Read the model definition and answer for the solid it produces. Units are mm, in the model's axes. Give positions to 0.01 mm unless a question says otherwise; leave off trailing zeros. Loops run counter-clockwise (first coordinate to the right, second up) from the corner with the lowest first, then second, coordinate; pieces in that order, holes last. Notation, with made-up numbers: (18.5, 64.5) -> (22.5, 64.5) arc R18 cw to (22.5, 79.5) -> close; hole circle Ø7 at (-6.5, 56.5). An arc over 180 degrees is marked (long way). One line per item, written item: value. Start each with the question number.
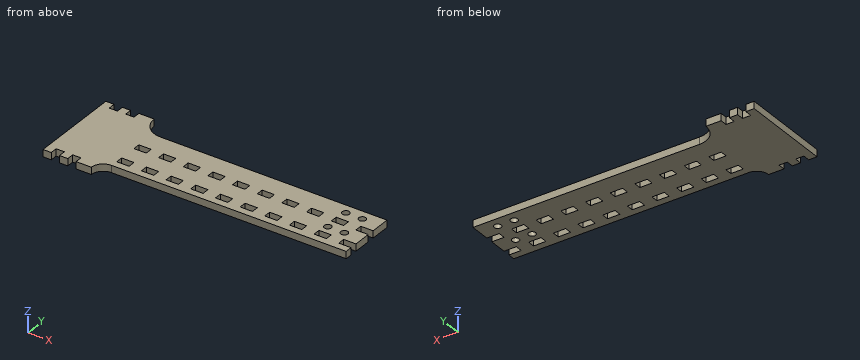
Autodesk Inventor part; units mm, degrees
ref_plane "YZ Plane" through (0, 0, 0) normal (1, 0, 0) x (0, 1, 0)
ref_plane "XZ Plane" through (0, 0, 0) normal (0, 1, 0) x (-1, 0, 0)
ref_plane "XY Plane" through (0, 0, 0) normal (0, 0, 1) x (1, 0, 0)
sketch "Sketch1" plane through (0, 0, 0) normal (0, 0, 1) x (1, 0, 0)
  line L0 (0, 0) -> (250, 0)
  line L1 (250, 0) -> (250, 77)
  line L2 (250, 77) -> (0, 77)
  line L3 (0, 77) -> (0, 0)
  dimension "d0" = 250
  dimension "d1" = 77
extrude "Extrusion1" add sketch "Sketch1" along normal blind 6
sketch "Sketch2" plane through (0, 0, 6) normal (0, 0, 1) x (1, 0, 0)
  line L0 (250, 77) -> (0, 77)
  line L1 (0, 77) -> (7, 77)
  line L2 (7, 77) -> (14, 77)
  line L3 (14, 77) -> (14, 71)
  line L4 (14, 71) -> (7, 71)
  line L5 (7, 71) -> (7, 77)
  line L6 (0, 0) -> (250, 0)
  line L7 (0, 0) -> (7, 0)
  line L8 (7, 0) -> (14, 0)
  line L9 (14, 0) -> (14, 6)
  line L10 (14, 6) -> (7, 6)
  line L11 (7, 6) -> (7, 0)
  dimension "d4" = 7
  dimension "d5" = 7
  dimension "d6" = 6
  dimension "d7" = 7
  dimension "d8" = 7
  dimension "d9" = 6
extrude "Extrusion2" cut sketch "Sketch2" against normal blind 6
pattern_linear "Rectangular Pattern1" count 2 spacing 14 along (1, 0, 0) of "Extrusion2"
sketch "Sketch3" plane through (0, 0, 6) normal (0, 0, 1) x (1, 0, 0)
  line L0 (250, 77) -> (28, 77)
  line L1 (41, 77) -> (49.5, 77)
  line L2 (28, 0) -> (250, 0)
  line L3 (41, 0) -> (51, 0)
  arc A0 (51, 10) -> (41, 0) centre (51, 0) ccw
  line L4 (41, 77) -> (58, 77)
  arc A1 (41, 77) -> (58, 60) centre (58, 77) ccw
  line L5 (58, 60) -> (250, 60)
  line L6 (51, 10) -> (250, 10)
  line L7 (250, 0) -> (250, 77)
  point P0 (0, 0)
  point P1 (0, 77)
  dimension "d15" = 41
  dimension "d21" = 34
extrude "Extrusion3" cut sketch "Sketch3" against normal blind 6
sketch "Sketch4" plane through (0, 0, 6) normal (0, 0, 1) x (1, 0, 0)
  line L0 (28, 0) -> (41, 0)
  line L1 (51.45, 16) -> (61.9, 16)
  line L2 (61.9, 16) -> (61.9, 22)
  line L3 (61.9, 22) -> (51.45, 22)
  line L4 (51.45, 22) -> (51.45, 16)
  line L5 (51.45, 37) -> (61.9, 37)
  line L6 (61.9, 37) -> (61.9, 43)
  line L7 (61.9, 43) -> (51.45, 43)
  line L8 (51.45, 43) -> (51.45, 37)
  point P0 (0, 0)
  point P1 (51, 10)
  dimension "d26" = 10.45
  dimension "d27" = 6
  dimension "d28" = 15
  dimension "d29" = 10.45
  dimension "d30" = 6
extrude "Extrusion4" cut sketch "Sketch4" against normal blind 6
pattern_linear "Rectangular Pattern2" count 10 spacing 20.9 along (1, 0, 0) of "Extrusion4"
sketch "Sketch5" plane through (0, 0, 6) normal (0, 0, 1) x (1, 0, 0)
  line L0 (250, 43) -> (250, 60)
  circle A0 centre (235, 51.5) radius 3
  circle A1 centre (221, 51.5) radius 3
  line L1 (250, 22) -> (250, 37)
  circle A2 centre (221, 29.5) radius 3
  circle A3 centre (235, 29.5) radius 3
  point P0 (0, 0)
  dimension "d37" = 6
  dimension "d39" = 6
  dimension "d40" = 6
  dimension "d41" = 6
extrude "Extrusion5" cut sketch "Sketch5" against normal blind 6
properties part number "g_arm1"
Item 1: Flat-ended cylindrical pins translate along their axes: pin 1 (1.8 mm diameter, centred on x = 184, z = 2.5, fed in from -Y); pin 2 (3 mm diameter, centred on x = 184.5, z = 1.5, fed in from +Y). Find the tip coordinate at first contact, or state that the pin passes through.
Item 2: Consider L1, parallel to Y at x = 221, z = 3.2; L2, parallel to Y at x = 162, z = 3.05; L3, parallel to Y at x = 235, z = 1.6. Determine where each line is inside the solid, lowest interval first. Write a range as [from, to].
Item 3: Section A-A, the plane y = 51.5 is taken. Determine the outline of the cut face in (x, z).
Item 4: Section B-B, the plane x = 235 is taken. Determine the outline of the cut face in (y, z), plus the area to 3 significant figures.
Item 5: Section D-D, the plane x = 45.5 is taken. Determine the outline of the cut face in (y, z), plus the area to 3 significant figures.
Item 6: Section C-C, the plane z = 1.7 is taken. State how many separate pieces and enclosed holes the cut face has, plus the area to 3 significant figures.
Computed values:
1. pin 1: y = 10
1. pin 2: y = 60
2. L1: [10, 16], [22, 26.5], [32.5, 37], [43, 48.5], [54.5, 60]
2. L2: [10, 16], [22, 37], [43, 60]
2. L3: [10, 26.5], [32.5, 48.5], [54.5, 60]
3. outline: (0, 0) -> (218, 0) -> (218, 6) -> (0, 6) -> close; (224, 0) -> (232, 0) -> (232, 6) -> (224, 6) -> close; (238, 0) -> (250, 0) -> (250, 6) -> (238, 6) -> close
4. outline: (10, 0) -> (26.5, 0) -> (26.5, 6) -> (10, 6) -> close; (32.5, 0) -> (48.5, 0) -> (48.5, 6) -> (32.5, 6) -> close; (54.5, 0) -> (60, 0) -> (60, 6) -> (54.5, 6) -> close
4. area: 228 mm²
5. outline: (8.35, 0) -> (65.48, 0) -> (65.48, 6) -> (8.35, 6) -> close
5. area: 343 mm²
6. separate pieces: 1
6. enclosed holes: 22
6. area: 12,200 mm²
